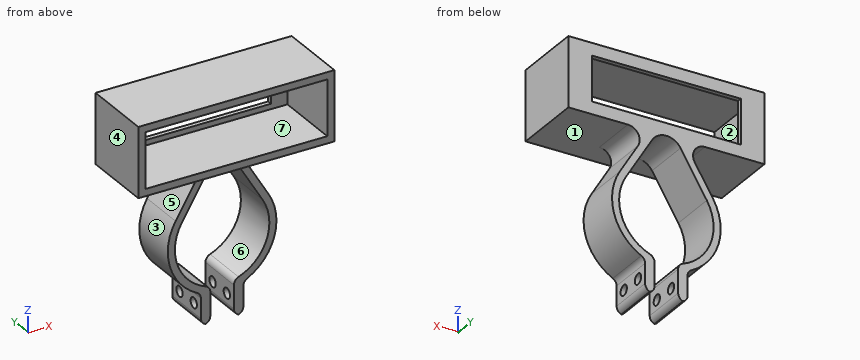
from build123d import *

# Parameters (mm, degrees)
F1_DEPTH    = 20
F3_DEPTH    = 20.001
F5_DEPTH    = 20
F6_T1_DEPTH = 20
F6_T3_DEPTH = 30.9947096091
F6_T5_DEPTH = 35
F7_W        = 83
F7_H        = 29.5
F7_W_2      = 77
F7_H_2      = 23.5
F8_DEPTH    = 30
F9_T1_DEPTH = 20
F10_R       = 2.2
F11_DEPTH   = 50.501
F12_W       = 77
F12_H       = 23.5
F12_W_2     = 63
F12_H_2     = 19
F13_DEPTH   = 2


# Not quite as in the source:
# - a fillet or chamfer that OpenCascade refuses, or shapes differently, is made with other operations: its cross-section is extruded or revolved along the edge and cut away or added


with BuildPart() as f1:
    # F0 (on Front) → F1 (new body)
    with BuildSketch(Plane.XZ):
        with BuildLine():
            ThreePointArc((8.5666506378, 30.3587301587), (0, 35.2), (-8.5666506378, 30.3587301587))
            Line((-8.5666506378, 30.3587301587), (-19.7032964668, 11.8650793651))
            ThreePointArc((-19.7032964668, 11.8650793651), (0, -23), (19.7032964668, 11.8650793651))
            Line((19.7032964668, 11.8650793651), (8.5666506378, 30.3587301587))
        make_face()
        with BuildLine():
            ThreePointArc((17.1333012755, 10.3174603175), (0, -20), (-17.1333012755, 10.3174603175))
            Line((-17.1333012755, 10.3174603175), (-5.9966554464, 28.8111111111))
            ThreePointArc((-5.9966554464, 28.8111111111), (0, 32.2), (5.9966554464, 28.8111111111))
            Line((5.9966554464, 28.8111111111), (17.1333012755, 10.3174603175))
        make_face(mode=Mode.SUBTRACT)
    extrude(amount=F1_DEPTH)

    # F2 (on face) → F3 (cut, through all)
    with BuildSketch(Plane.XZ.offset(20)):
        with BuildLine():
            ThreePointArc((5, -19.364916731), (0, -20), (-5, -19.364916731))
            Line((-5, -19.364916731), (-5, -22.4499443206))
            ThreePointArc((-5, -22.4499443206), (0, -23), (5, -22.4499443206))
            Line((5, -22.4499443206), (5, -19.364916731))
        make_face()
    extrude(amount=-F3_DEPTH, mode=Mode.SUBTRACT)

    # F4 (on Front) → F5 (join, through all)
    with BuildSketch(Plane.XZ):
        Polygon((-5, -34.4499443206), (-5, -22.4499443206), (-9, -21.1660104885), (-9, -34.4499443206), align=None)
        Polygon((5, -34.4499443206), (9, -34.4499443206), (9, -21.1660104885), (5, -22.4499443206), align=None)
    extrude(amount=F5_DEPTH)

    # F6: fillet of radius 3 on 8 edges, made by hand

    # F6_s2 → F6_t1 (join)
    with BuildSketch(Plane.XZ):
        with BuildLine():
            ThreePointArc((-9, -23.0651251893), (-9.4354487572, -21.5085016244), (-10.6153846154, -20.4037645906))
            ThreePointArc((-10.6153846154, -20.4037645906), (-9.8150946559, -20.8005749174), (-9, -21.1660104885))
            Line((-9, -21.1660104885), (-9, -23.0651251893))
        make_face()
        with BuildLine():
            ThreePointArc((9, -23.0651251893), (9.4354487572, -21.5085016244), (10.6153846154, -20.4037645906))
            ThreePointArc((10.6153846154, -20.4037645906), (9.8150946559, -20.8005749174), (9, -21.1660104885))
            Line((9, -21.1660104885), (9, -23.0651251893))
        make_face()
    extrude(amount=F6_T1_DEPTH)

    # F6_s4 → F6_t3 (cut)
    with BuildSketch(Plane.XZ.offset(-5.4973548045)):
        with BuildLine():
            ThreePointArc((-5, -21.5638586528), (-5.5372337928, -19.8507379307), (-6.9565217391, -18.7511814373))
            ThreePointArc((-6.9565217391, -18.7511814373), (-5.9861315369, -19.0831399204), (-5, -19.364916731))
            Line((-5, -19.364916731), (-5, -21.5638586528))
        make_face()
        with BuildLine():
            ThreePointArc((5, -21.5638586528), (5.5372337928, -19.8507379307), (6.9565217391, -18.7511814373))
            ThreePointArc((6.9565217391, -18.7511814373), (5.9861315369, -19.0831399204), (5, -19.364916731))
            Line((5, -19.364916731), (5, -21.5638586528))
        make_face()
    extrude(amount=F6_T3_DEPTH, mode=Mode.SUBTRACT)

    # F6_s6 → F6_t5 (cut)
    with BuildSketch(Plane.XZ.offset(-7.5)):
        with BuildLine():
            ThreePointArc((-8, -34.4499443206), (-5.8786796564, -33.5712646642), (-5, -31.4499443206))
            Line((-5, -31.4499443206), (-5, -34.4499443206))
            Line((-5, -34.4499443206), (-8, -34.4499443206))
        make_face()
        with BuildLine():
            ThreePointArc((5, -31.4499443206), (5.8786796564, -33.5712646642), (8, -34.4499443206))
            Line((8, -34.4499443206), (5, -34.4499443206))
            Line((5, -34.4499443206), (5, -31.4499443206))
        make_face()
        with BuildLine():
            ThreePointArc((6, -34.4499443206), (8.1213203436, -33.5712646642), (9, -31.4499443206))
            Line((9, -31.4499443206), (9, -34.4499443206))
            Line((9, -34.4499443206), (6, -34.4499443206))
        make_face()
        with BuildLine():
            ThreePointArc((-9, -31.4499443206), (-8.1213203436, -33.5712646642), (-6, -34.4499443206))
            Line((-6, -34.4499443206), (-9, -34.4499443206))
            Line((-9, -34.4499443206), (-9, -31.4499443206))
        make_face()
    extrude(amount=F6_T5_DEPTH, mode=Mode.SUBTRACT)

    # F7 (on Front) → F8 (join)
    with BuildSketch(Plane.XZ):
        with Locations((0, 46.95)):
            Rectangle(F7_W, F7_H)
        with Locations((0, 46.95)):
            Rectangle(F7_W_2, F7_H_2, mode=Mode.SUBTRACT)
    extrude(amount=F8_DEPTH)

    # F9: fillet of radius 5 on 2 edges, made by hand

    # F9_s2 → F9_t1 (join)
    with BuildSketch(Plane.XZ):
        with BuildLine():
            ThreePointArc((-16.3053853354, 32.2), (-11.9524078833, 29.659997419), (-12.0220600165, 24.6206349206))
            Line((-12.0220600165, 24.6206349206), (-11.5937274846, 24.3626984127))
            ThreePointArc((-11.5937274846, 24.3626984127), (-8.1383181059, 30.1007936508), (-6.7843570071, 31.85))
            Line((-6.7843570071, 31.85), (-7.1414284285, 32.7))
            Line((-7.1414284285, 32.7), (-16.3053853354, 32.7))
            Line((-16.3053853354, 32.7), (-16.3053853354, 32.2))
        make_face()
        with BuildLine():
            ThreePointArc((16.3053853354, 32.2), (11.9524078833, 29.659997419), (12.0220600165, 24.6206349206))
            Line((12.0220600165, 24.6206349206), (11.5937274846, 24.3626984127))
            ThreePointArc((11.5937274846, 24.3626984127), (8.1383181059, 30.1007936508), (6.7843570071, 31.85))
            Line((6.7843570071, 31.85), (7.1414284285, 32.7))
            Line((7.1414284285, 32.7), (16.3053853354, 32.7))
            Line((16.3053853354, 32.7), (16.3053853354, 32.2))
        make_face()
    extrude(amount=F9_T1_DEPTH)

    # F10 (on face) → F11 (cut, through all)
    with BuildSketch(Plane(origin=(-9, 0, 0), x_dir=(0, -1, 0), z_dir=(-1, 0, 0))):
        with Locations((5, -27.257534755)):
            Circle(F10_R)
        with Locations((15, -27.257534755)):
            Circle(F10_R)
    extrude(amount=-F11_DEPTH, mode=Mode.SUBTRACT)

    # F12 (on Front) → F13 (join)
    with BuildSketch(Plane.XZ):
        with Locations((0, 46.95)):
            Rectangle(F12_W, F12_H)
        with Locations((0, 46.95)):
            Rectangle(F12_W_2, F12_H_2, mode=Mode.SUBTRACT)
    extrude(amount=F13_DEPTH)


solid = f1.part
Design review of the part built by this model. Coordinates are the model's own, in mm. Face numbers are marked on the shaded views. A direction names the side the tool comes from. Give positions to 0.01 mm unless a question says otherwise; leave off trailing zeros. Loops run counter-clockwise (first coordinate to the right, second up) from the corner with the lowest first, then second, coordinate; pieces in that order, holes last. Notation, with made-up numbers: (53, 89.25) - (93, 89.25) arc R24 ccw to (93, 124.25) - close; hole circle Ø11 at (59.25, 34.25). An arc over 180 degrees is marked (long way). Use CSV: the item, a comma, the result in double quotes. Start each with the question number.
1. Wall thickness on L1, parallel to Z at x = 38, y = -4.5; L2, parallel to X at y = -25.5, z = 48; L3, parallel to Z at x = -7.7, y = -15: over which ranges is each line inside the solid? List them lowest first.
2. Add section A-A (x = 36.5). State the section outline as (y, z) points.
3. Add section C-C (y = -15). Count the separate pieces of the cut face and the enclosed holes in it, plus the area to 3 significant figures.
4. Add section D-D (x = -2). State the section outline as (y, z) points, plus the area to 3 significant figures.
5. Insertion check: P1, Ø5, axis at y = -5, z = -27.26, coming from the +X side; P2, Ø3, axis at x = -16.5, y = -9.5, coming from the -Z side; P3, Ø11, axis at y = -15, z = -27.5, coming from the -X side. Each pin has a flat end and moves straight along its axis. Give the tip position at first contact, or say it passes through.
6. Add section B-B (z = 7). State the section outline as (x, y) points (3 decimals).
7. Machinability: for the marked faces 4, 5, 6 and 7, which of the approach directions +Z, -Z, +X, -X, +Y, -Y give a long, thin tool a straight path to every point of the face, cutting with its end or side? Answer none if there is none.
8. Draft analysis for pull direction X (two halves, no side actions). For the marked faces 1, 2 and 3, state which applies: released by +X, released by -X, zero draft, split by the parting line, or undercut.
Results found:
1,L1,"z = 32.2 to 35.2, 58.7 to 61.7"
1,L2,"x = -41.5 to -38.5, 38.5 to 41.5"
1,L3,"z = -33.92 to -29.46, -25.06 to -18.46, 25.98 to 35.2, 58.7 to 61.7"
2,outline,"(-30, 32.2) - (0, 32.2) - (0, 61.7) - (-30, 61.7) - (-30, 58.7) - (-2, 58.7) - (-2, 35.2) - (-30, 35.2) - close"
3,separate pieces,"3"
3,enclosed holes,"1"
3,area,"1,130 mm²"
4,outline,"(-30, 32.2) - (-20, 32.2) - (-20, 31.91) - (0, 31.91) - (0, 37.45) - (-2, 37.45) - (-2, 35.2) - (-30, 35.2) - close; (-30, 58.7) - (-2, 58.7) - (-2, 56.45) - (0, 56.45) - (0, 61.7) - (-30, 61.7) - close"
4,area,"195 mm²"
5,P1,"stops at x = 9"
5,P2,"stops at z = -17.44"
5,P3,"stops at x = -9.2"
6,outline,"(-21.909, -20) - (-18.735, -20) - (-18.735, 0) - (-21.909, 0) - close; (18.735, -20) - (21.909, -20) - (21.909, 0) - (18.735, 0) - close"
7,face 4,"+Z, -Z, -X, +Y, -Y"
7,face 5,"-X, +Y, -Y"
7,face 6,"+Y, -Y"
7,face 7,"-Y"
8,face 1,"zero draft"
8,face 2,"undercut"
8,face 3,"released by -X"
